For this review, take the finished solid that the model builds, in its own axes (mm). Face numbers are marked on the shaded views. A direction names the side the tool comes from. Give positions to 0.01 mm unless a question says otherwise; leave off trailing zeros. Write each loop counter-clockwise with the first axis right and the second up, starting at its lowest first coordinate (ties: lowest second). Pieces come first, ordered by that corner, then holes. Notation, with made-up numbers: M -24.5,38 L 27.5,38 A12 ccw 27.5,61 Z; hole C 55,-3.75 d4. An arc over 180 degrees is marked long. Use one line per item in the form item = value. Start each with the question number.
Q1. For probe 1 along Y at (x, z) = (-102, 9); probe 2 along Y at (x, z) = (-103.35, 44.46); probe 3 along Y at (x, z) = (-103.6, 79.46), list the stretches that pass through material, from the lowest coordinate up. Write a range as [from, to].
Q2. Consider section C-C on y = 12.85. Write out the cut boundary in (x, z), and give its area (3 significant figures).
Q3. Consider section B-B on x = 70. Write out the cut boundary in (y, z).
Q4. Consider section D-D on z = 154.5. Write out the cut boundary in (x, y).
Q5. Clearance check with flat-ended pins moving along their axes: pin 1 Ø5 at (x, y) = (74.5, 19.5) entering from -Z; pin 2 Ø3.5 at (y, z) = (41.83, 44.46) entering from -X; pin 3 Ø6 at (y, z) = (57, 154) entering from +X. State where each tip first meets the part, or that it passes through.
Q6. Consider section A-A on z = 44.46. Write out the cut boundary in (x, y), and give its area (3 significant figures).
Q7. Tool access review of the marked faces 1, 2 and 3: name each direction out of +Z, -Z, +X, -X, +Y, -Y from which nothing blocks a thin tool from reaching the whole face with its end or side.
```python
from build123d import *

# Parameters (mm, degrees)
SKETCH1_W                 = 210
SKETCH1_H                 = 145
BOSS_EXTRUDE1_DEPTH       = 180
SKETCH9_W                 = 201
SKETCH9_H                 = 145
CUT_EXTRUDE4_DEPTH        = 15.5
SKETCH2_R                 = 42.5
CUT_EXTRUDE1_DEPTH        = 25
SKETCH3_R                 = 52.5
CUT_EXTRUDE2_DEPTH        = 5.2
SKETCH4_R                 = 16
CUT_EXTRUDE3_DEPTH        = 5
FILLET1_R                 = 30
SHELL1_START              = 25.7
SHELL1_DEPTH              = 149.3
SHELL1_START_2            = 20.5
SHELL1_2_DEPTH            = 5.2
M6_TAPPED_HOLE1_D         = 5
M6_TAPPED_HOLE1_DEPTH     = 10
M6_TAPPED_HOLE1_TIP       = 1.502151548
F_6_0MM_DOWEL_HOLE1_D     = 6
F_6_0MM_DOWEL_HOLE1_DEPTH = 13
F_6_0MM_DOWEL_HOLE1_TIP   = 1.802581857
FILLET2_R                 = 10


# Read off the part's stored shape, not the designer's step: Shell1
with BuildPart() as part:
    # Sketch1 → Boss-Extrude1 (new body)
    with BuildSketch(Plane.XY):
        Rectangle(SKETCH1_W, SKETCH1_H)
    extrude(amount=BOSS_EXTRUDE1_DEPTH)

    # Sketch9 → Cut-Extrude4 (cut)
    with BuildSketch(Plane(origin=(0, 0, 0), x_dir=(-1, 0, 0), z_dir=(0, 0, -1))):
        with Locations((-4.5, 0)):
            Rectangle(SKETCH9_W, SKETCH9_H)
    extrude(amount=-CUT_EXTRUDE4_DEPTH, mode=Mode.SUBTRACT)

    # Sketch2 → Cut-Extrude1 (cut)
    with BuildSketch(Plane(origin=(0, 0, 0), x_dir=(-1, 0, 0), z_dir=(0, 0, -1))):
        with Locations((31.5, 12.85)):
            Circle(SKETCH2_R)
    extrude(amount=-CUT_EXTRUDE1_DEPTH, mode=Mode.SUBTRACT)

    # Sketch3 → Cut-Extrude2 (cut)
    with BuildSketch(Plane(origin=(0, 0, 15.5), x_dir=(-1, 0, 0), z_dir=(0, 0, -1))):
        with Locations((31.5, 12.85)):
            Circle(SKETCH3_R)
    extrude(amount=-CUT_EXTRUDE2_DEPTH, mode=Mode.SUBTRACT)

    # Sketch4 → Cut-Extrude3 (cut)
    with BuildSketch(Plane.ZY.offset(105)):
        with Locations((44.46, -15.32)):
            Circle(SKETCH4_R)
    extrude(amount=-CUT_EXTRUDE3_DEPTH, mode=Mode.SUBTRACT)

    # Fillet1
    fillet1_edges = [part.edges().sort_by_distance(p)[0] for p in [
        (105, -72.5, 97.75),
        (105, 72.5, 97.75),
    ]]
    fillet(fillet1_edges, radius=FILLET1_R)

    # Shell1 outline → Shell1 (cut)
    with BuildSketch(Plane.XY.offset(SHELL1_START)):
        with BuildLine():
            Line((-100, -67.5), (75, -67.5))
            ThreePointArc((75, -67.5), (92.67766953, -60.17766953), (100, -42.5))
            Line((100, -42.5), (100, 42.5))
            ThreePointArc((100, 42.5), (92.67766953, 60.17766953), (75, 67.5))
            Line((75, 67.5), (-100, 67.5))
            Line((-100, 67.5), (-100, -67.5))
        make_face()
    extrude(amount=SHELL1_DEPTH, mode=Mode.SUBTRACT)

    # Shell1 2 outline → Shell1 2 (cut)
    with BuildSketch(Plane.XY.offset(SHELL1_START_2)):
        with BuildLine():
            Line((-100, 67.5), (-100, -67.5))
            Line((-100, -67.5), (75, -67.5))
            ThreePointArc((75, -67.5), (92.67766953, -60.17766953), (100, -42.5))
            Line((100, -42.5), (100, 42.5))
            ThreePointArc((100, 42.5), (92.67766953, 60.17766953), (75, 67.5))
            Line((75, 67.5), (-13.621870903, 67.5))
            ThreePointArc((-13.621870903, 67.5), (-31.5, -44.65), (-49.378129097, 67.5))
            Line((-49.378129097, 67.5), (-100, 67.5))
        make_face()
    extrude(amount=SHELL1_2_DEPTH, mode=Mode.SUBTRACT)

    # M6 Tapped Hole1
    with Locations(Plane.ZY.offset(105)):
        with Locations((9.46, 41.83), (79.46, 41.83), (79.46, -53.42), (9.46, -53.42)):
            Hole(M6_TAPPED_HOLE1_D / 2, depth=M6_TAPPED_HOLE1_DEPTH)
            with Locations((0, 0, -(M6_TAPPED_HOLE1_DEPTH + M6_TAPPED_HOLE1_TIP / 2))):  # 118° drill point
                Cone(0, M6_TAPPED_HOLE1_D / 2, M6_TAPPED_HOLE1_TIP, mode=Mode.SUBTRACT)

    # Ø6.0mm Dowel Hole1
    with Locations(Plane.ZY.offset(105)):
        with Locations((44.46, 41.83), (44.46, -53.42)):
            Hole(F_6_0MM_DOWEL_HOLE1_D / 2, depth=F_6_0MM_DOWEL_HOLE1_DEPTH)
            with Locations((0, 0, -(F_6_0MM_DOWEL_HOLE1_DEPTH + F_6_0MM_DOWEL_HOLE1_TIP / 2))):  # 118° drill point
                Cone(0, F_6_0MM_DOWEL_HOLE1_D / 2, F_6_0MM_DOWEL_HOLE1_TIP, mode=Mode.SUBTRACT)

    # Fillet2
    # the kernel refuses this fillet: 10 mm, written as the material it takes off along each edge
    with BuildSketch(Plane(origin=(-130, -72.5, 180), x_dir=(0, 0, -1), z_dir=(1, 0, 0))) as fillet2_piece_1:
        with BuildLine():
            CenterArc((FILLET2_R, FILLET2_R), FILLET2_R, 180, 90)
            Line((0, FILLET2_R), (0, 0))
            Line((0, 0), (FILLET2_R, 0))
        make_face()
    extrude(amount=205, mode=Mode.SUBTRACT)
    with BuildSketch(Plane(origin=(75, 72.5, 15.5), x_dir=(0, -1, 0), z_dir=(-1, 0, 0))) as fillet2_piece_2:
        with BuildLine():
            CenterArc((FILLET2_R, FILLET2_R), FILLET2_R, 180, 90)
            Line((0, FILLET2_R), (0, 0))
            Line((0, 0), (FILLET2_R, 0))
        make_face()
    extrude(amount=171, mode=Mode.SUBTRACT)
    with BuildSketch(Plane(origin=(105, -42.5, 15.5), x_dir=(-1, 0, 0), z_dir=(0, 1, 0))) as fillet2_piece_3:
        with BuildLine():
            CenterArc((FILLET2_R, FILLET2_R), FILLET2_R, 180, 90)
            Line((0, FILLET2_R), (0, 0))
            Line((0, 0), (FILLET2_R, 0))
        make_face()
    extrude(amount=85, mode=Mode.SUBTRACT)
    with BuildSketch(Plane(origin=(105, -42.5, 180), x_dir=(-1, 0, 0), z_dir=(0, 1, 0))) as fillet2_piece_4:
        with BuildLine():
            CenterArc((FILLET2_R, -FILLET2_R), FILLET2_R, 90, 90)
            Line((0, -FILLET2_R), (0, 0))
            Line((0, 0), (FILLET2_R, 0))
        make_face()
    extrude(amount=85, mode=Mode.SUBTRACT)
    with BuildSketch(Plane(origin=(-96, -72.5, 15.5), x_dir=(0, 0, 1), z_dir=(1, 0, 0))) as fillet2_piece_5:
        with BuildLine():
            CenterArc((FILLET2_R, -FILLET2_R), FILLET2_R, 90, 90)
            Line((0, -FILLET2_R), (0, 0))
            Line((0, 0), (FILLET2_R, 0))
        make_face()
    extrude(amount=171, mode=Mode.SUBTRACT)
    with BuildSketch(Plane(origin=(75, 42.5, 15.5), x_dir=(1, 0, 0), z_dir=(0, -1, 0))) as fillet2_piece_6:
        with BuildLine():
            CenterArc((30 - FILLET2_R, FILLET2_R), FILLET2_R, 270, 90)
            Line((30, FILLET2_R), (30, 0))
            Line((30, 0), (30 - FILLET2_R, 0))
        make_face()
    revolve(axis=Axis((75, 42.5, 15.5), (0, 0, 1)), revolution_arc=90, mode=Mode.SUBTRACT)
    with BuildSketch(Plane(origin=(75, -42.5, 15.5), x_dir=(0, -1, 0), z_dir=(-1, 0, 0))) as fillet2_piece_7:
        with BuildLine():
            CenterArc((30 - FILLET2_R, FILLET2_R), FILLET2_R, 270, 90)
            Line((30, FILLET2_R), (30, 0))
            Line((30, 0), (30 - FILLET2_R, 0))
        make_face()
    revolve(axis=Axis((75, -42.5, 15.5), (0, 0, 1)), revolution_arc=90, mode=Mode.SUBTRACT)
    with BuildSketch(Plane(origin=(75, 72.5, 180), x_dir=(0, -1, 0), z_dir=(-1, 0, 0))) as fillet2_piece_8:
        with BuildLine():
            CenterArc((FILLET2_R, -FILLET2_R), FILLET2_R, 90, 90)
            Line((0, -FILLET2_R), (0, 0))
            Line((0, 0), (FILLET2_R, 0))
        make_face()
    extrude(amount=205, mode=Mode.SUBTRACT)
    with BuildSketch(Plane(origin=(75, 42.5, 180), x_dir=(1, 0, 0), z_dir=(0, -1, 0))) as fillet2_piece_9:
        with BuildLine():
            CenterArc((30 - FILLET2_R, -FILLET2_R), FILLET2_R, 0, 90)
            Line((30, -FILLET2_R), (30, 0))
            Line((30, 0), (30 - FILLET2_R, 0))
        make_face()
    revolve(axis=Axis((75, 42.5, 180), (0, 0, 1)), revolution_arc=90, mode=Mode.SUBTRACT)
    with BuildSketch(Plane(origin=(75, -42.5, 180), x_dir=(0, -1, 0), z_dir=(-1, 0, 0))) as fillet2_piece_10:
        with BuildLine():
            CenterArc((30 - FILLET2_R, -FILLET2_R), FILLET2_R, 0, 90)
            Line((30 - FILLET2_R, 0), (30, 0))
            Line((30, 0), (30, -FILLET2_R))
        make_face()
    revolve(axis=Axis((75, -42.5, 180), (0, 0, 1)), revolution_arc=90, mode=Mode.SUBTRACT)


solid = part.part
```
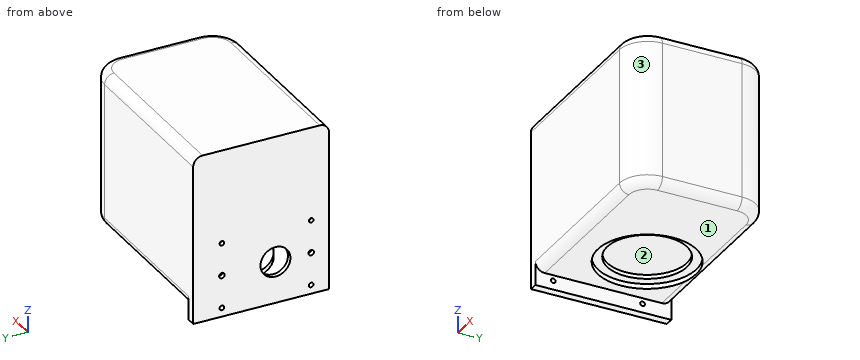
Working result:
q1.probe_1 = [-72.5, -55.88], [-50.96, 39.37], [44.29, 72.5]
q1.probe_2 = [-72.5, -56.42], [-50.42, -31.32], [0.68, 38.83], [44.83, 72.5]
q1.probe_3 = [-72.5, -55.92], [-50.92, 39.33], [44.33, 72.5]
q2.outline = M -105,0 L -96,0 L -96,15.5 L -84,15.5 L -84,20.7 L -74,20.7 L -74,25 L 11,25 L 11,20.7 L 21,20.7 L 21,15.5 L 95,15.5 A10 ccw 105,25.5 L 105,170 A10 ccw 95,180 L -105,180 Z; hole M -100,20.5 L -89,20.5 L -89,25.7 L 26,25.7 L 26,20.5 L 100,20.5 L 100,175 L -100,175 Z
q2.area = 3,430 mm²
q3.outline = M -72.5,25.5 A10 ccw -62.5,15.5 L 62.5,15.5 A10 ccw 72.5,25.5 L 72.5,170 A10 ccw 62.5,180 L -62.5,180 A10 ccw -72.5,170 Z; hole M -67.5,20.5 L 67.5,20.5 L 67.5,175 L -67.5,175 Z
q4.outline = M -105,-72.5 L 75,-72.5 A30 ccw 105,-42.5 L 105,42.5 A30 ccw 75,72.5 L -105,72.5 Z; hole M -100,-67.5 L 75,-67.5 A25 ccw 100,-42.5 L 100,42.5 A25 ccw 75,67.5 L -100,67.5 Z
q5.pin_1 = 15.5
q5.pin_2 = 99.98
q5.pin_3 = 102.71
q6.outline = M -105,-72.5 L 75,-72.5 A30 ccw 105,-42.5 L 105,42.5 A30 ccw 75,72.5 L -105,72.5 L -105,44.83 L -100,44.83 L -100,67.5 L 75,67.5 A25 cw 100,42.5 L 100,-42.5 A25 cw 75,-67.5 L -100,-67.5 L -100,-56.42 L -105,-56.42 Z; M -105,-50.42 L -100,-50.42 L -100,-31.32 L -105,-31.32 Z; M -105,0.68 L -100,0.68 L -100,38.83 L -105,38.83 Z
q6.area = 3,110 mm²
q7.face_1 = -Z, +X, +Y, -Y
q7.face_2 = -Z
q7.face_3 = +Z, -Z, +X, -Y
